Source: CAD feature listing. Evaluate the final solid. Frame: model axes, mm. A direction names the side the tool comes from. Round coordinates to 2 decimals unless told otherwise and drop trailing zeros. Write each loop counter-clockwise with the first axis right and the second up, starting at its lowest first coordinate (ties: lowest second). Pieces come first, ordered by that corner, then holes.
```python
from build123d import *

# Parameters (mm, degrees)
BOSS_EXTRUDE1_DEPTH                     = 54.37886
CUT_EXTRUDE1_DEPTH                      = 87.700652431
CUT_EXTRUDE1_DEPTH_BACK                 = 87.700652431
SKETCH2_R                               = 4.7625
CBORE_FOR_M6_HEX_HEAD_BOLT1_D           = 6.6
CBORE_FOR_M6_HEX_HEAD_BOLT1_DEPTH       = 14.019159957
CBORE_FOR_M6_HEX_HEAD_BOLT1_CBORE_D     = 15
CBORE_FOR_M6_HEX_HEAD_BOLT1_CBORE_DEPTH = 4.38
CBORE_FOR_M6_HEX_HEAD_BOLT1_TIP         = 1.982840043


with BuildPart() as part:
    # Sketch1 → Boss-Extrude1 (new body)
    with BuildSketch(Plane(origin=(0, 0, 0), x_dir=(1, 0, 0), z_dir=(0, 1, 0))):
        Polygon((15.630864679, -74.497263655), (15.630864679, -35.611217769), (60.611215954, -35.611217769), (61.693150972, -41.86836701), (29.545852981, -47.427014582), (29.545852981, -68.383645943), (65.211603651, -62.21661634), (66.293538669, -68.47376558), (31.457873152, -74.497263655), align=None)
    extrude(amount=BOSS_EXTRUDE1_DEPTH)

    # Sketch2 → Cut-Extrude1 (cut, two sides: drawn at the far end of the back side and taken through both)
    with BuildSketch(Plane(origin=(13.420740042, 0, 77.616097039), x_dir=(0.9853778331324855, 0, -0.17038346742312627), z_dir=(0.17038346742312627, 0, 0.9853778331324856)).offset(-CUT_EXTRUDE1_DEPTH_BACK)):
        with Locations((35.981087332, 27.18943)):
            Circle(SKETCH2_R)
        Polygon((30.711163119, 0), (53.657385878, 17.02943), (53.657385878, 0), align=None)
        Polygon((53.657385878, 37.34943), (30.711163119, 54.37886), (53.657385878, 54.37886), align=None)
    extrude(amount=CUT_EXTRUDE1_DEPTH + CUT_EXTRUDE1_DEPTH_BACK, mode=Mode.SUBTRACT)

    # CBORE for M6 Hex Head Bolt1
    with Locations(Plane(origin=(29.545852981, 0, 0), x_dir=(0, 0, -1), z_dir=(1, 0, 0))):
        with Locations((-55.447263655, 14.48943), (-55.447263655, 39.88943)):
            CounterBoreHole(CBORE_FOR_M6_HEX_HEAD_BOLT1_D / 2, CBORE_FOR_M6_HEX_HEAD_BOLT1_CBORE_D / 2, CBORE_FOR_M6_HEX_HEAD_BOLT1_CBORE_DEPTH, depth=CBORE_FOR_M6_HEX_HEAD_BOLT1_DEPTH)
            with Locations((0, 0, -(CBORE_FOR_M6_HEX_HEAD_BOLT1_DEPTH + CBORE_FOR_M6_HEX_HEAD_BOLT1_TIP / 2))):  # 118° drill point
                Cone(0, CBORE_FOR_M6_HEX_HEAD_BOLT1_D / 2, CBORE_FOR_M6_HEX_HEAD_BOLT1_TIP, mode=Mode.SUBTRACT)


solid = part.part
```
Q1. Set-up query: faces 4 (the face through (29.546, 27, 60)), 5 (the face through (27, 0, 55)), 6 (the face through (38.701, 26.809, 45.844)). Return all of +Z, -Z, +X, -X, +Y, -Y with unobstructed straight access to the full face (end or side cutting, diameter ignored); none if empty.
Q2. Section query A-A, the plane z = 55. Output: boundary loops of the cut face in (x, y).
Q3. Section query C-C, the plane y = 26. Output: boundary loops of the cut face in (x, z).
Q4. Line query: line 1 (X direction, y = 46, z = 62); line 2 (Y direction, x = 29, z = 53.5); line 3 (X direction, y = 33, z = 53.5). Output: solid intervals per line, ascending.
Q5. Section query D-D, the plane y = 15.5. Output: boundary loops of the cut face in (x, z), and give its area (3 significant figures).
Q6. Mould query, pull axis Z, two halves, no side actions, for faces 1 (the face through (39.203, 26.809, 66.714)), 2 (the face through (54.281, 8.396, 67.284)), 3 (the face through (24, 27, 74.497)). Classes: pulls with the +Z half, pulls with the -Z half, needs draft (parallel to the pull), parting line crosses it, or undercut.
Q7. Section query B-B, the plane x = 32.5. Output: boundary loops of the cut face in (y, z).
Q8. Pin query (flat end, axial travel): P1, Ø10, axis at x = 41.5, y = 40.5, coming from the +Z side; P2, Ø6.5, axis at y = 24, z = 56.5, coming from the +X side; P3, Ø4.5, axis at y = 17.5, z = 56.5, coming from the +X side. Return the tip coordinate at first contact, or that it passes through.
Filled in:
1. face 4: +Y, -Y
1. face 5: +Z, -Z, +X, -X, -Y
1. face 6: +X, +Y, -Y
2. outline: (15.63, 0) - (29.55, 0) - (29.55, 7) - (25.17, 7) - (25.17, 11.22) - (15.63, 11.22) - close; (15.63, 17.76) - (25.17, 17.76) - (25.17, 21.98) - (29.55, 21.98) - (29.55, 32.4) - (25.17, 32.4) - (25.17, 36.62) - (15.63, 36.62) - close; (15.63, 43.16) - (25.17, 43.16) - (25.17, 47.38) - (29.55, 47.38) - (29.55, 54.38) - (15.63, 54.38) - close
3. outline: (15.63, 35.61) - (37.99, 35.61) - (39.73, 45.67) - (29.55, 47.43) - (29.55, 68.38) - (43.25, 66.01) - (44.33, 72.27) - (31.46, 74.5) - (15.63, 74.5) - close; (47.35, 35.61) - (60.61, 35.61) - (61.69, 41.87) - (48.82, 44.09) - close; (52.34, 64.44) - (65.21, 62.22) - (66.29, 68.47) - (53.42, 70.7) - close
4. line 1: x = 15.63 to 29.55
4. line 2: y = 0 to 7.25, 21.73 to 32.65, 47.13 to 54.38
4. line 3: x = 15.63 to 25.17
5. outline: (15.63, 35.61) - (58.52, 35.61) - (59.66, 42.22) - (29.55, 47.43) - (29.55, 48.02) - (25.17, 48.02) - (25.17, 52.31) - (15.63, 52.31) - close; (15.63, 58.59) - (25.17, 58.59) - (25.17, 62.88) - (29.55, 62.88) - (29.55, 68.38) - (63.18, 62.57) - (64.26, 68.82) - (31.46, 74.5) - (15.63, 74.5) - close
5. area: 910 mm2
6. face 1: undercut
6. face 2: pulls with the -Z half
6. face 3: pulls with the +Z half
7. outline: (0, 35.61) - (54.38, 35.61) - (54.38, 46.92) - (0, 46.92) - close; (0, 67.87) - (54.38, 67.87) - (54.38, 74.32) - (0, 74.32) - close
8. P1: stops at z = 73.63
8. P2: stops at x = 29.55
8. P3: stops at x = 25.17
